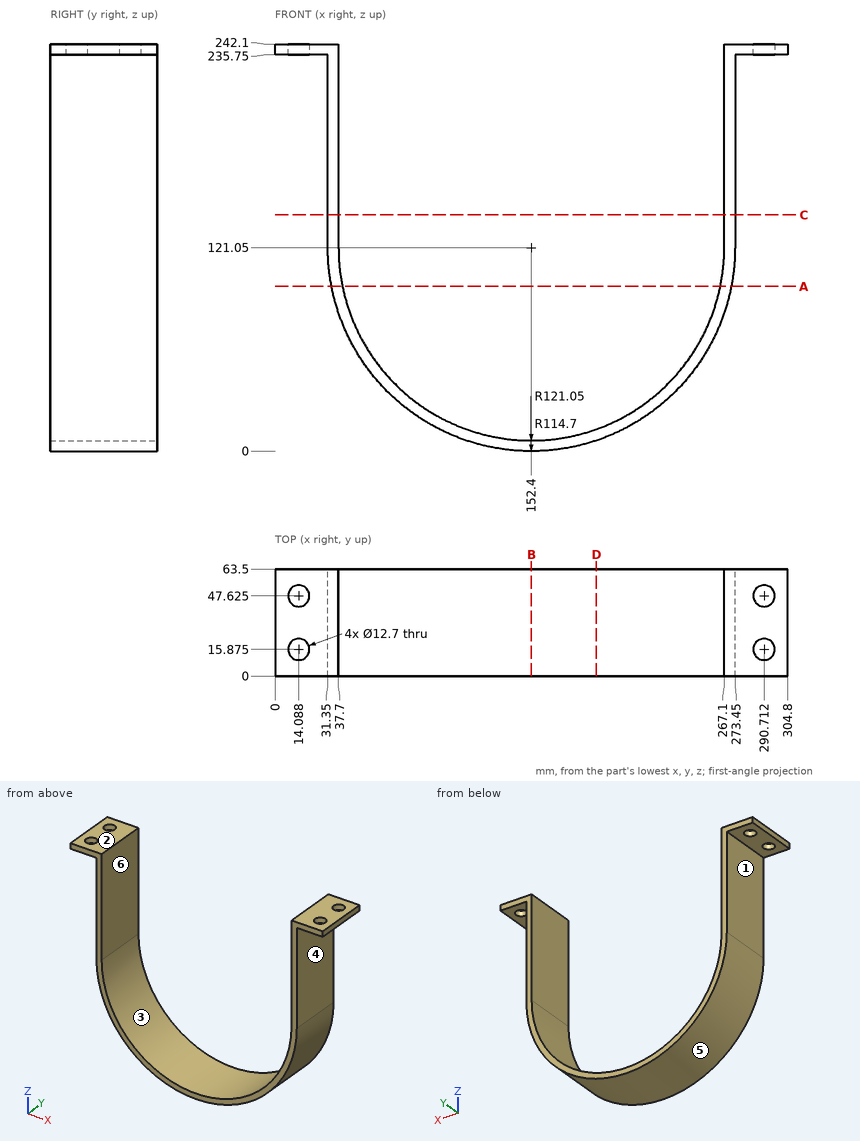
Input: dimensioned drawing with shaded views. Units: mm. Origin: part minimum x, y, z. A direction names the side the tool comes from. Coordinates: 2 decimals unless noted, no trailing zeros. Loops run counter-clockwise (first coordinate to the right, second up) from the corner with the lowest first, then second, coordinate; pieces in that order, holes last. Notation, with made-up numbers: M 30.25,81 L 73.25,81 A32 ccw 73.25,113 Z; hole C 49.5,-36 d10. An arc over 180 degrees is marked long. Use a Markdown table: item, result. Add a question column.
Q1. Section query C-C, the plane z = 140.5. Return loops of the section in (x, y).
Q2. Material intervals for L1, parallel to X at y = 7, z = 214.5; L2, parallel to X at y = 47, z = 38 (1 decimal); L3, parallel to Z at x = 278.5, y = 47, sorted ascending.
Q3. Section query D-D, the plane x = 191. Return loops of the section in (y, z), and give its area (3 significant figures).
Q4. Draft query along X for the marked faces 1, 2 and 3. Return one class per face: pulls with the +X half, pulls with the -X half, needs draft (parallel to the pull), parting line crosses it, or undercut.
Q5. Section query A-A, the plane z = 98. Return loops of the section in (x, y) (1 decimal).
Q6. Section query B-B, the plane x = 152.4. Return loops of the section in (y, z).
Q7. First-contact query: pin 1 (3 mm diameter, centred on y = 26.5, z = 65, fed in from -X); pin 2 (12 mm diameter, centred on y = 27, z = 164.5, fed in from +X); pin 3 (16.5 mm diameter, centred on x = 14.09, y = 47.62, fed in from +Z); pin 4 (2 mm diameter, centred on y = 22, z = 68.5, fed in from -X) (1 decimal). Flat tips, straight axial feed; report the tip coordinate or a pass-through.
Q8. Access query for the marked faces 4, 5 and 6. Directions: +Z, -Z, +X, -X, +Y, -Y. A direction counts if a zero-diameter tool reaches every point of the face in a straight line with its end or side. Return the directions, or none.
Result:
| question | item | result |
|---|---|---|
| 1 | outline | M 31.35,0 L 37.7,0 L 37.7,63.5 L 31.35,63.5 Z; M 267.1,0 L 273.45,0 L 273.45,63.5 L 267.1,63.5 Z |
| 2 | L1 | x = 31.35 to 37.7, 267.1 to 273.45 |
| 2 | L2 | x = 64.3 to 73.3, 231.5 to 240.5 |
| 2 | L3 | z = 235.75 to 242.1 |
| 3 | outline | M 0,6.32 L 63.5,6.32 L 63.5,13.04 L 0,13.04 Z |
| 3 | area | 427 mm2 |
| 4 | face 1 | pulls with the -X half |
| 4 | face 2 | needs draft |
| 4 | face 3 | undercut |
| 5 | outline | M 33.6,0 L 40,0 L 40,63.5 L 33.6,63.5 Z; M 264.8,0 L 271.2,0 L 271.2,63.5 L 264.8,63.5 Z |
| 6 | outline | M 0,0 L 63.5,0 L 63.5,6.35 L 0,6.35 Z |
| 7 | pin 1 | stops at x = 44.34 |
| 7 | pin 2 | stops at x = 273.45 |
| 7 | pin 3 | stops at z = 242.1 |
| 7 | pin 4 | stops at x = 42.9 |
| 8 | face 4 | -Z, +X, +Y, -Y |
| 8 | face 5 | -Z, +Y, -Y |
| 8 | face 6 | +Z, +Y, -Y |
